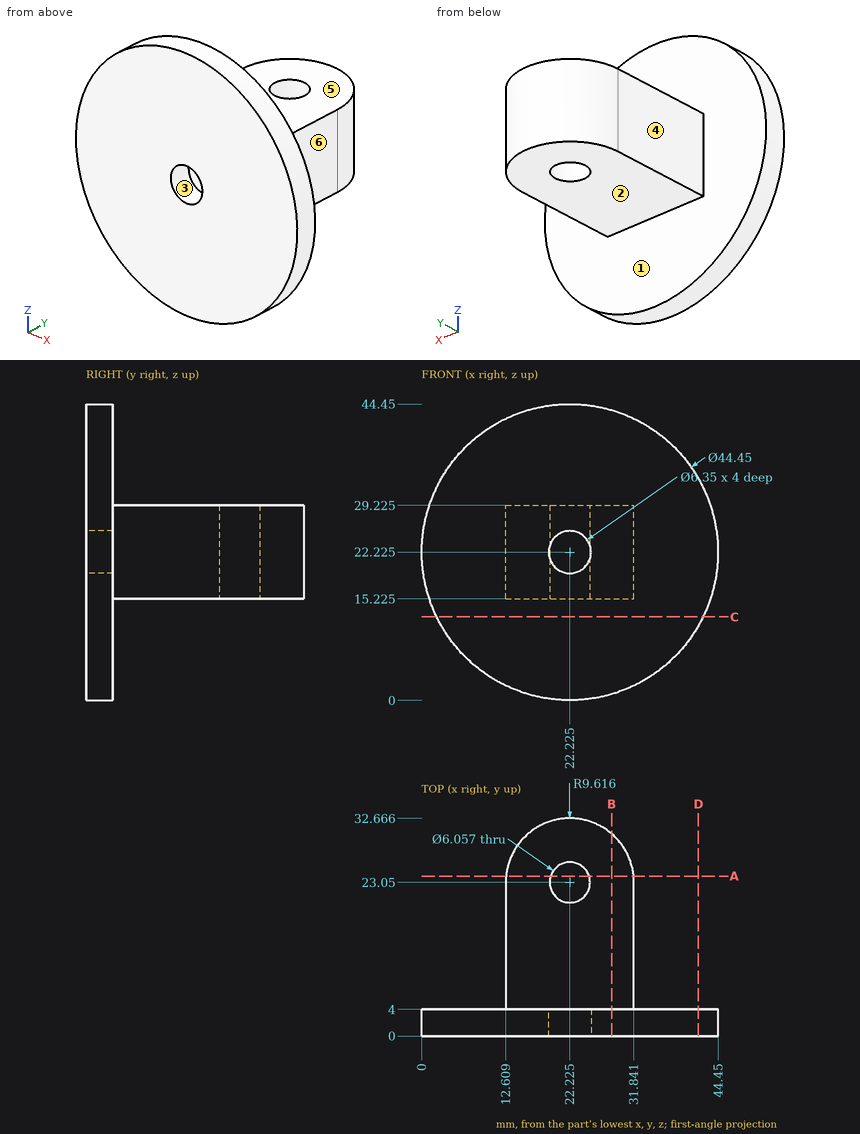
Job drawing, mm, ordinate dimensions from the low corner. One solid piece. A direction names the side the tool comes from. Coordinates: 2 decimals unless noted, no trailing zeros. Order: outer loops, then holes, each group sorted by start corner. A loop starts at its lowest first (then second) coordinate and runs counter-clockwise, first axis right, second up. Notation, with made-up numbers: (-29.5, -2.75) - (12.5, -2.75) arc R23 ccw to (12.5, 6.25) - close; hole circle Ø11 at (89.25, -24.5). An arc over 180 degrees is marked (long way). Return JSON: item names as keys, results as strings. Group by question number.
1) Tool access for the marked faces 4, 5 and 6: list every direction of +Z, -Z, +X, -X, +Y, -Y with a clear straight run to the whole face (end or side of a thin tool).
2) Saw through at D-D, the plane x = 41.5. Write the cut outline in (y, z).
3) Saw through at B-B, the plane x = 28.5. Write the cut outline in (y, z) (1 decimal).
4) Saw through at C-C, the plane z = 12.5. Write the cut outline in (x, y).
5) Probe line 1 (X direction, y = 23, z = 24); line 2 (Y direction, x = 32, z = 33.5); line 3 (Z direction, x = 25, y = 19) (1 decimal). List the from-to ranges inside material, lowest first. Write a range as from..to.
6) Mould opens along Z. For the marked faces 1, 2 and 3 say: released by +Z, released by -Z, zero draft, split by the parting line, or undercut.
7) Saw through at A-A, the plane y = 24. Write the cut outline in (x, z) (1 decimal).
8) Flat gauge pins, fed straight in: P1, Ø2, axis at x = 26.5, z = 14.5, coming from the +Y side; P2, Ø1, axis at x = 37.5, z = 8.5, coming from the +Y side; P3, Ø11, axis at y = 11, z = 20, coming from the -X side. Where does each tip first touch, or does it go through?
Values found:
{
 "1": {"face 4": "+Z, -Z, -X, +Y", "face 5": "+Z, +X, -X, +Y", "face 6": "+Z, -Z, +X, +Y"},
 "2": {"outline": "(0, 11.16) - (4, 11.16) - (4, 33.29) - (0, 33.29) - close"},
 "3": {"outline": "(0, 0.9) - (4, 0.9) - (4, 15.2) - (30.3, 15.2) - (30.3, 29.2) - (4, 29.2) - (4, 43.5) - (0, 43.5) - close"},
 "4": {"outline": "(2.24, 0) - (42.21, 0) - (42.21, 4) - (2.24, 4) - close"},
 "5": {"line 1": "x = 12.61..19.2, 25.25..31.84", "line 2": "y = 0..4", "line 3": "z = 15.2..29.2"},
 "6": {"face 1": "zero draft", "face 2": "released by -Z", "face 3": "undercut"},
 "7": {"outline": "(12.7, 15.2) - (19.3, 15.2) - (19.3, 29.2) - (12.7, 29.2) - close; (25.1, 15.2) - (31.8, 15.2) - (31.8, 29.2) - (25.1, 29.2) - close"},
 "8": {"P1": "stops at y = 31.97", "P2": "stops at y = 4", "P3": "stops at x = 12.61"}
}
